Autodesk Fusion 360 part; units mm, degrees
ref_plane "WorkPlane3" through (54.5653, 17.8993, 37.432) normal (0, 1, 0) x (-1, 0, 0)
sketch "Top part base" plane through (54.5653, 17.8993, 37.432) normal (0, 1, 0) x (1, 0, 0)
  line L0 (25.2893, -113.3578) -> (25.2893, -39.0578)
  line L1 (25.2893, -39.0578) -> (-19.7107, -44.2645)
  line L2 (-19.7107, -44.2645) -> (-19.7107, -102.7645)
  line L3 (-19.7107, -102.7645) -> (25.2893, -113.3578)
  line L4 (-30, 0) -> (100, 0) construction
  dimension "d112" = 45
  dimension "d113" = 58.5
  dimension "d114" = 74.3
  dimension "d115" = 6.6
extrude "Extrude9" add sketch "Top part base" along normal blind 2
sketch "Anchor" plane through (0, 17.8993, 0) normal (0, -1, 0) x (1, 0, 0)
  line L0 (79.8546, 150.7899) -> (34.8546, 140.1965)
  line L1 (34.8546, 140.1965) -> (34.8546, 81.6965)
  line L2 (34.8546, 81.6965) -> (79.8546, 76.4899)
  line L3 (79.8546, 76.4899) -> (79.8546, 150.7899)
  line L4 (11.5702, 84.3906) -> (87.0208, 75.6607) construction
  line L5 (46.7751, 80.3173) -> (66.6426, 78.0185)
  line L6 (66.6426, 78.0185) -> (69.516, 102.8529)
  line L7 (69.516, 102.8529) -> (49.6485, 105.1516)
  line L8 (49.6485, 105.1516) -> (46.7751, 80.3173)
  dimension "d86" = 90
  dimension "d87" = 90
  dimension "d88" = 90
  dimension "d89" = 12
  dimension "d90" = 20
  dimension "d91" = 25
extrude "Extrude10" add sketch "Anchor" along normal blind 14 contours L2 L5 L6 L7 L8
sketch "Stopper battery" plane through (0, 17.8993, 0) normal (0, -1, 0) x (1, 0, 0)
  line L0 (69.516, 102.8529) -> (66.6426, 78.0185)
  line L1 (66.6426, 78.0185) -> (79.8546, 76.4899)
  line L2 (79.8546, 76.4899) -> (79.8546, 150.7899)
  line L3 (79.8546, 150.7899) -> (34.8546, 140.1965)
  line L4 (34.8546, 140.1965) -> (34.8546, 81.6965)
  line L5 (34.8546, 81.6965) -> (46.7751, 80.3173)
  line L6 (46.7751, 80.3173) -> (49.6485, 105.1516)
  line L7 (49.6485, 105.1516) -> (69.516, 102.8529)
  line L8 (34.8546, 140.1965) -> (72.8169, 149.1331)
  line L9 (34.8546, 140.1965) -> (42.3018, 108.5613)
  line L10 (42.3018, 108.5613) -> (76.3705, 116.5813)
  line L11 (76.3705, 116.5813) -> (76.1414, 117.5547)
  line L12 (76.1414, 117.5547) -> (43.0461, 109.7638)
  line L13 (43.0461, 109.7638) -> (36.0572, 139.4523)
  line L14 (36.0572, 139.4523) -> (72.0727, 147.9306)
  line L15 (72.8169, 149.1331) -> (75.5667, 137.4524)
  line L16 (75.5667, 137.4524) -> (74.5933, 137.2233)
  line L17 (74.5933, 137.2233) -> (72.0727, 147.9306)
  dimension "d116" = 39
  dimension "d117" = 32.5
  dimension "d118" = 35
  dimension "d119" = 1
  dimension "d120" = 1
  dimension "d121" = 1
  dimension "d122" = 12
  dimension "d123" = 1
  dimension "d124" = 1
sketch "Anchor hole" plane through (9.7882, 0, 84.5968) normal (-0.1149, 0, -0.9934) x (0, 1, 0)
  line L0 (17.8993, 70.5339) -> (17.8993, 57.2337)
  line L1 (17.8993, 57.2337) -> (3.8993, 57.2337)
  line L2 (3.8993, 57.2337) -> (3.8993, 37.2337)
  line L3 (3.8993, 37.2337) -> (17.8993, 37.2337)
  line L4 (17.8993, 37.2337) -> (17.8993, 25.2337)
  line L5 (17.8993, 25.2337) -> (19.8993, 25.2337)
  line L6 (19.8993, 25.2337) -> (19.8993, 70.5339)
  line L7 (19.8993, 70.5339) -> (17.8993, 70.5339)
  circle A0 centre (10.8993, 47.2337) radius 4
  line L8 (19.8993, 47.2337) -> (3.8993, 47.2337) construction
  dimension "d109" = 8
  dimension "d110" = 7
hole "Hole3" at (56.7088, 10.8993, 79.1679) direction (0.1149, 0, 0.9934) diameter 8 depth 20 tip angle 118
extrude "Extrude12" add sketch "Stopper battery" along normal blind 6 contours L3 L8 L9 L10 L11 L12 L13 L14 L15 L16 L17
sketch "Strap holes" plane through (0, 17.8993, 0) normal (0, -1, 0) x (1, 0, 0)
  line L0 (72.8169, 149.1331) -> (75.5667, 137.4524)
  line L1 (75.5667, 137.4524) -> (74.5933, 137.2233)
  line L2 (74.5933, 137.2233) -> (72.0727, 147.9306)
  line L3 (72.0727, 147.9306) -> (36.0572, 139.4523)
  line L4 (36.0572, 139.4523) -> (43.0461, 109.7638)
  line L5 (43.0461, 109.7638) -> (76.1414, 117.5547)
  line L6 (76.1414, 117.5547) -> (76.3705, 116.5813)
  line L7 (76.3705, 116.5813) -> (42.3018, 108.5613)
  line L8 (42.3018, 108.5613) -> (34.8546, 140.1965)
  line L9 (34.8546, 140.1965) -> (34.8546, 81.6965)
  line L10 (34.8546, 81.6965) -> (46.7751, 80.3173)
  line L11 (46.7751, 80.3173) -> (49.6485, 105.1516)
  line L12 (49.6485, 105.1516) -> (69.516, 102.8529)
  line L13 (69.516, 102.8529) -> (66.6426, 78.0185)
  line L14 (66.6426, 78.0185) -> (79.8546, 76.4899)
  line L15 (79.8546, 76.4899) -> (79.8546, 150.7899)
  line L16 (79.8546, 150.7899) -> (72.8169, 149.1331)
  line L17 (34.8546, 104.4899) -> (37.8546, 104.4899)
  line L18 (37.8546, 104.4899) -> (37.8546, 84.4899)
  line L19 (37.8546, 84.4899) -> (34.8546, 84.4899)
  line L20 (34.8546, 84.4899) -> (34.8546, 104.4899)
  line L21 (76.8546, 104.4899) -> (79.8546, 104.4899)
  line L22 (79.8546, 104.4899) -> (79.8546, 84.4899)
  line L23 (79.8546, 84.4899) -> (76.8546, 84.4899)
  line L24 (76.8546, 84.4899) -> (76.8546, 104.4899)
  dimension "d127" = 20
  dimension "d128" = 8
  dimension "d129" = 3
extrude "Extrude13" cut sketch "Strap holes" against normal blind 10 contours L15 L21 L22 L23 L24 | L9 L17 L18 L19 L20
fillet "Fillet5" radius 3 4 edges at (59.5823, 3.8993, 104.0022) (68.0793, 3.8993, 90.4357) (48.2118, 3.8993, 92.7344) (56.7088, 3.8993, 79.1679)
Can you work these out from the model? Positions are in its coordinate system, mm. A direction names the side the tool comes from. Round coordinates to 2 decimals unless told otherwise and drop trailing zeros. Loops run counter-clockwise (first coordinate to the right, second up) from the corner with the lowest first, then second, coordinate; pieces in that order, holes last. Notation, with made-up numbers: (50.25, 59.5) - (70.25, 59.5) arc R22 ccw to (70.25, 96.5) - close; hole circle Ø9 at (88, 39). An arc over 180 degrees is marked (long way). Answer in a Markdown table with one row per item. Add a question column.
Q1. I want a section at A-A on y = 16. List the corners of the cut face in (x, z) for me.
Q2. I need wall thicknesses on L1, parallel to X at y = 8, z = 81; L2, parallel to Z at x = 71, y = 17.25; L3, parallel to Y at x = 77, z = 137. Which ranges of each line are inside material? Lowest first, please.
Q3. Which directions (+Z, -Z, +X, -X, +Y, -Y) give clear straight access to the entire face, cutting with the end or side of a thin tool? Please do faces 1 (the flat face through (73.35, 14.94, 142.5)), 2 (the flat face through (78, 19, 104.49)), 3 (the conical face through (58.97, 11.54, 101.04)).
Q4. I want a section at C-C on x = 45.5. List the corners of the cut face in (y, z) for me, and give its area (3 significant figures).
Q5. I want a section at D-D on z = 132. List the corners of the cut face in (x, y) for me, and give its area (3 significant figures).
Q6. We'd pull the mould along Z, two halves only. Please class faces 4 (the flat face through (47.8, 11.899, 142.5)), 5 (the flat face through (38.526, 14.941, 124.6)), 6 (the flat face through (59.098, 14.941, 112.515)): pulls with the +Z half, pulls with the -Z half, needs draft (parallel to the pull), parting line crosses it, or undercut.
Q7. For pin 1 Ø2 at (x, y) = (59.5, 10.5) entering from +Z; pin 2 Ø2 at (y, z) = (19, 94.5) entering from -X; pin 3 Ø1 at (y, z) = (19, 95) entering from +X; pin 4 Ø6 at (y, z) = (6.5, 126) entering from -X, each with a flat end and sliding along its axis, tell me the tip position at first contact or that it passes through.
Q8. I want a section at B-B on z = 141.5. List the corners of the cut face in (x, y) for me.
A:
| question | item | result |
|---|---|---|
| 1 | outline | (34.85, 140.2) - (42.3, 108.56) - (76.37, 116.58) - (76.14, 117.55) - (43.05, 109.76) - (36.06, 139.45) - (72.07, 147.93) - (74.59, 137.22) - (75.57, 137.45) - (72.82, 149.13) - close; (46.78, 80.32) - (66.64, 78.02) - (69.52, 102.85) - (49.65, 105.15) - close |
| 2 | L1 | 46.85 to 54.15, 59.69 to 66.99 |
| 2 | L2 | 115.32 to 116.34, 147.68 to 148.71 |
| 2 | L3 | 17.9 to 19.9 |
| 3 | face 1 | -Y |
| 3 | face 2 | +X, +Y, -Y |
| 3 | face 3 | none |
| 4 | outline | (11.9, 109.31) - (17.9, 109.31) - (17.9, 80.46) - (19.9, 80.46) - (19.9, 142.7) - (11.9, 142.7) - (11.9, 141.68) - (17.9, 141.68) - (17.9, 110.34) - (11.9, 110.34) - close |
| 4 | area | 137 mm^2 |
| 5 | outline | (34.85, 17.9) - (36.78, 17.9) - (36.78, 11.9) - (37.81, 11.9) - (37.81, 17.9) - (79.85, 17.9) - (79.85, 19.9) - (34.85, 19.9) - close |
| 5 | area | 96.2 mm^2 |
| 6 | face 4 | needs draft |
| 6 | face 5 | pulls with the -Z half |
| 6 | face 6 | undercut |
| 7 | pin 1 | z = 104.13 |
| 7 | pin 2 | x = 37.85 |
| 7 | pin 3 | x = 76.85 |
| 7 | pin 4 | through |
| 8 | outline | (40.39, 11.9) - (44.76, 11.9) - (44.76, 17.9) - (73.59, 17.9) - (73.59, 11.9) - (74.61, 11.9) - (74.61, 17.9) - (79.85, 17.9) - (79.85, 19.9) - (40.39, 19.9) - close |
